```python
from build123d import *

# Parameters (mm, degrees)
F1_DEPTH = 1850
F3_DEPTH = 25
F5_DEPTH = 25


with BuildPart() as f1:
    # F0 (on Front) → F1 (new body)
    with BuildSketch(Plane.XZ):
        with BuildLine():
            Line((0, 1), (0, 19))
            Line((0, 19), (-1, 19))
            Line((-1, 19), (-1, 1))
            ThreePointArc((-1, 1), (-0.4142135624, -0.4142135624), (1, -1))
            Line((1, -1), (248, -1))
            Line((248, -1), (248, -2))
            Line((248, -2), (239, -2))
            Line((239, -2), (239, -3))
            Line((239, -3), (248, -3))
            ThreePointArc((248, -3), (248.7071067812, -2.7071067812), (249, -2))
            Line((249, -2), (249, -1))
            ThreePointArc((249, -1), (248.7071067812, -0.2928932188), (248, 0))
            Line((248, 0), (1, 0))
            ThreePointArc((1, 0), (0.2928932188, 0.2928932188), (0, 1))
        make_face()
    extrude(amount=-F1_DEPTH)

    # F2 (on face) → F3 (cut, symmetric)
    with BuildSketch(Plane.XY):
        Polygon((249, -77.7916684747), (249, 0), (-151, 400), (-151, 0), (-141.1382748954, -77.7916684747), align=None)
    extrude(amount=F3_DEPTH, both=True, mode=Mode.SUBTRACT)

    # F4 (on face) → F5 (cut, symmetric)
    with BuildSketch(Plane.XY):
        Polygon((0, 1893.902085615), (0, 1850), (456.097914385, 1393.902085615), (456.097914385, 1893.902085615), align=None)
    extrude(amount=F5_DEPTH, both=True, mode=Mode.SUBTRACT)


solid = f1.part
```
Geometry check sheet. Reference: the model listing, model coordinates, mm. A direction names the side the tool comes from. Give positions to 0.01 mm unless a question says otherwise; leave off trailing zeros. Order: outer loops, then holes, each group sorted by start corner. A loop starts at its lowest first (then second) coordinate and runs counter-clockwise, first axis right, second up. Notation, with made-up numbers: (-39.5, 33) - (-31.5, 33) arc R18 ccw to (-31.5, 64) - close; hole circle Ø7 at (-28, -22.5). An arc over 180 degrees is marked (long way). Answer in a Markdown table with one row per item. Add a question column.
Q1. Cross-section at B-B, the plane z = 9.75. Enter the section's corners in (x, y).
Q2. Gauge pin test, flat ends, axial feed: pin 1 (2.5 mm diameter, centred on x = 242.5, y = 874.5, fed in from +Z); pin 2 (10 mm diameter, centred on x = 194, z = 0.5, fed in from -Y); pin 3 (9 mm diameter, centred on y = 868.5, z = 13.5, fed in from +X). Record the tip position at first contact, or that the pin passes through.
Q3. Cross-section at C-C, the plane x = 45.5. Enter the section's corners in (y, z).
Q4. Tool access check on faces 1 (the flat face through (126, 912, 0)), 2 (the flat face through (123.9, 1726.1, -0.5)). Record the directions out of +Z, -Z, +X, -X, +Y, -Y that give a thin tool (end or side, any length) a straight path to the whole face; none if there is none.
Q5. Cross-section at A-A, the plane y = 605. Enter the section's corners in (x, z).
Q6. Material ranges on probe 1 along X at (y, z) = (1533, 14.5); probe 2 along X at (y, z) = (663.5, -0.5), recorded low to high. Write a range as from..to.
Check values:
| question | item | result |
|---|---|---|
| 1 | outline | (-1, 250) - (0, 249) - (0, 1850) - (-1, 1850) - close |
| 2 | pin 1 | stops at z = 0 |
| 2 | pin 2 | stops at y = 50.03 |
| 2 | pin 3 | stops at x = 0 |
| 3 | outline | (203.5, -1) - (1804.5, -1) - (1804.5, 0) - (203.5, 0) - close |
| 4 | face 1 | +Z, +X, +Y, -Y |
| 4 | face 2 | +Z, -Z, +X, +Y |
| 5 | outline | (-1, 1) arc R2 ccw to (1, -1) - (248, -1) - (248, -2) - (239, -2) - (239, -3) - (248, -3) arc R1 ccw to (249, -2) - (249, -1) arc R1 ccw to (248, 0) - (1, 0) arc R1 cw to (0, 1) - (0, 19) - (-1, 19) - close |
| 6 | probe 1 | x = -1..0 |
| 6 | probe 2 | x = -0.32..248.87 |
